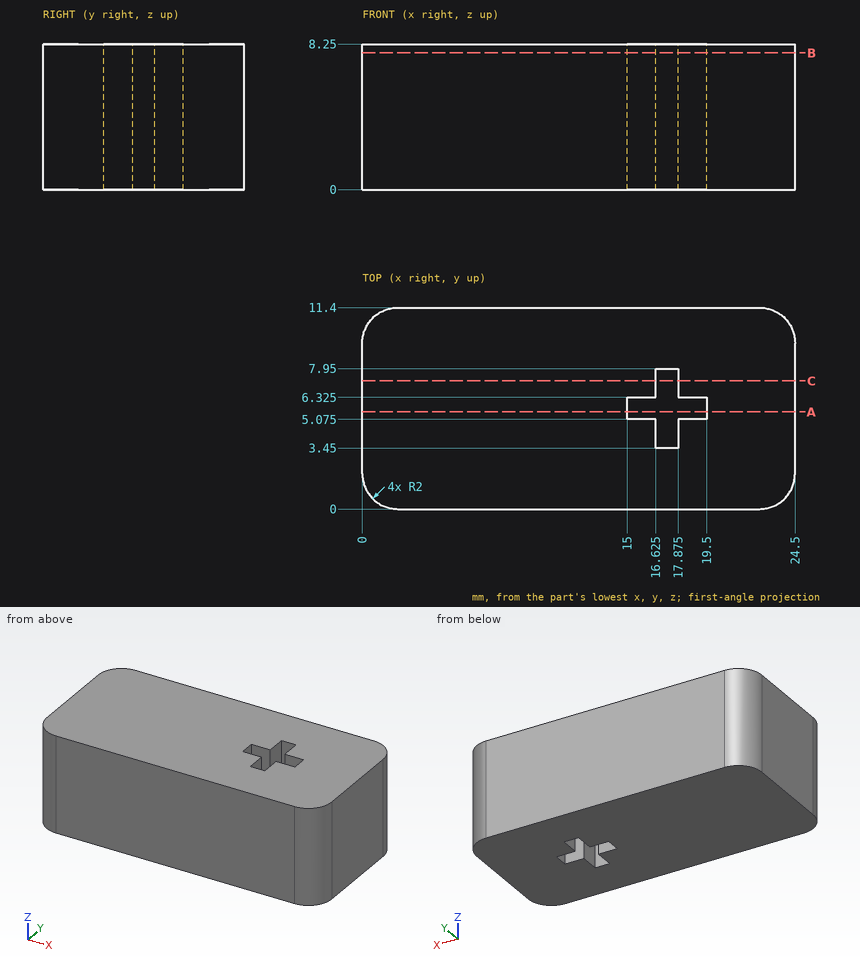
Design review of the part shown in the three views and the two pictorial views. Dimensions are in mm from the part's minimum x, y and z. Coordinates: 2 decimals unless noted, no trailing zeros. Order: outer loops, then holes, each group sorted by start corner. A loop starts at its lowest first (then second) coordinate and runs counter-clockwise, first axis right, second up.
1) Take a section at C-C, the plane y = 7.25. Give the boundary of the cut face in (x, z) (3 decimals).
2) Take a section at A-A, the plane y = 5.5. Give the boundary of the cut face in (x, z), and give its area (3 significant figures).
3) Take a section at B-B, the plane z = 7.75. Give the boundary of the cut face in (x, y) (3 decimals), and give its area (3 significant figures).
4) Wall thickness on line 1 along X through (y, z) = (4.5, 3) (3 decimals); line 2 along Y through (x, z) = (17, 6.75); line 3 along Y through (x, z) = (15.5, 2.75) (3 decimals): over which ranges is each line inside the solid? List them lowest first.
Returned:
1. outline: (0, 0) - (16.625, 0) - (16.625, 8.25) - (0, 8.25) - close; (17.875, 0) - (24.5, 0) - (24.5, 8.25) - (17.875, 8.25) - close
2. outline: (0, 0) - (15, 0) - (15, 8.25) - (0, 8.25) - close; (19.5, 0) - (24.5, 0) - (24.5, 8.25) - (19.5, 8.25) - close
2. area: 165 mm2
3. outline: (0, 2) arc R2 ccw to (2, 0) - (22.5, 0) arc R2 ccw to (24.5, 2) - (24.5, 9.4) arc R2 ccw to (22.5, 11.4) - (2, 11.4) arc R2 ccw to (0, 9.4) - close; hole (15, 5.075) - (16.625, 5.075) - (16.625, 3.45) - (17.875, 3.45) - (17.875, 5.075) - (19.5, 5.075) - (19.5, 6.325) - (17.875, 6.325) - (17.875, 7.95) - (16.625, 7.95) - (16.625, 6.325) - (15, 6.325) - close
3. area: 266 mm2
4. line 1: x = 0 to 16.625, 17.875 to 24.5
4. line 2: y = 0 to 3.45, 7.95 to 11.4
4. line 3: y = 0 to 5.075, 6.325 to 11.4
